Can you work these out from the model? Positions are in its coordinate system, mm. Face numbers are marked on the shaded views. A direction names the side the tool comes from. Coordinates: 2 decimals unless noted, no trailing zeros. Write each loop counter-clockwise with the first axis right and the second up, starting at its lowest first coordinate (ties: lowest second). Pieces come first, ordered by that corner, then holes. Notation, with made-up numbers: (14, 1) - (25, 1) arc R22 cw to (25, 21) - close; hole circle Ø1 at (-15, -21.5). An arc over 180 degrees is marked (long way). One line per question, with ' | ' between items. Start each with the question number.
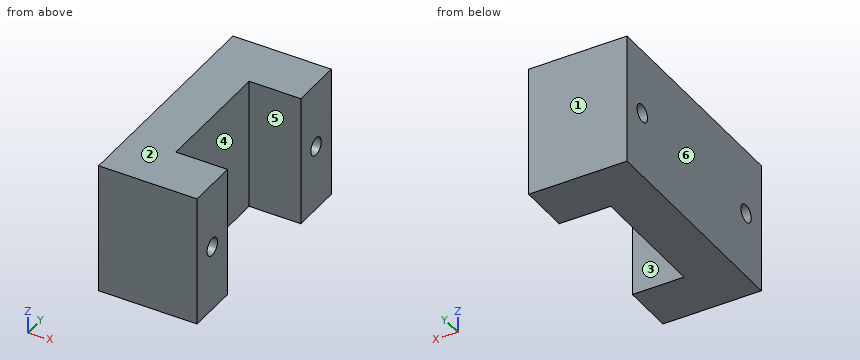
Autodesk Inventor part; units mm, degrees
ref_plane "YZ Plane" through (0, 0, 0) normal (1, 0, 0) x (0, 1, 0)
ref_plane "XZ Plane" through (0, 0, 0) normal (0, 1, 0) x (-1, 0, 0)
ref_plane "XY Plane" through (0, 0, 0) normal (0, 0, 1) x (1, 0, 0)
sketch "Sketch1" plane through (0, 0, 0) normal (1, 0, 0) x (0, 1, 0)
  line L0 (22.6064, 29.4791) -> (-21.3864, 29.4791)
  line L1 (-21.3864, 29.4791) -> (-21.3864, 4.0791)
  line L2 (-21.3864, 4.0791) -> (22.6064, 4.0791)
  line L3 (22.6064, 4.0791) -> (22.6064, 29.4791)
  point P0 (0, 0)
  dimension "d0" = 43.9928
  dimension "d1" = 25.4
extrude "Extrusion1" add sketch "Sketch1" along normal blind 19.05
sketch "Sketch2" plane through (19.05, 0, 0) normal (1, 0, 0) x (0, 0, -1)
  line L0 (-29.4791, 22.6064) -> (-29.4791, -21.3864)
  line L1 (-29.4791, -21.3864) -> (-4.0791, -21.3864)
  line L2 (-4.0791, 22.6064) -> (-29.4791, 22.6064)
  point P0 (0, 0)
  point P1 (-16.7791, 17.6064)
  point P2 (-16.7791, -16.3864)
  dimension "d4" = 0
  dimension "d5" = 12.7
  dimension "d6" = 5
  dimension "d7" = 5
hole "Hole1" at (19.05, 17.6064, 16.7791) at (19.05, -16.3864, 16.7791) direction (-1, 0, 0) diameter 3.4036 end through all
sketch "Sketch3" plane through (0, -21.3864, 29.4791) normal (0, 0, 1) x (1, 0, 0)
  line L0 (19.05, 10) -> (9.05, 10)
  line L1 (9.05, 10) -> (9.05, 33.9928)
  line L2 (9.05, 33.9928) -> (19.05, 33.9928)
  line L3 (19.05, 33.9928) -> (19.05, 10)
  line L4 (19.05, 43.9928) -> (19.05, 0)
  line L5 (0, 43.9928) -> (19.05, 43.9928)
  line L6 (0, 0) -> (19.05, 0)
  point P0 (0, 21.3864)
  dimension "d15" = 0
  dimension "d16" = 10
  dimension "d17" = 10
  dimension "d18" = 10
extrude "Extrusion2" cut sketch "Sketch3" against normal blind 60.325
properties part number "LidarV4MountBack"
(1) If we mould it in two halves opening along Y, with no side actions, what happens to the marked faces 1, 2, 3 and 4? For each: +Y half, -Y half, draft (parallel to the pull), parting line (faces both ways), or undercut.
(2) Which directions (+Z, -Z, +X, -X, +Y, -Y) give clear straight access to the entire face, cutting with the end or side of a thin tool? Please do the marked faces 5 and 6.
(3) If we section it at A-A on x = 16.5: List the corners of the cut face in (y, z) for me.
(4) I'm going to push flat-ended pins straight in: pin 1 (2 mm diameter, centred on y = -3, z = 17, fed in from +X); pin 2 (3 mm diameter, centred on y = 9.5, z = 13.5, fed in from -X); pin 3 (2 mm diameter, centred on y = 17.61, z = 16.78, fed in from +X). Where does each tip first touch, or does it pass through?
(5) If we section it at C-C on z = 6.5: List the corners of the cut face in (x, y) for me, plus the area to 3 significant figures.
(6) If I drill on probe 1 along Y at (x, z) = (18.25, 13.5); probe 2 along Z at (x, y) = (15.75, 17.5); probe 3 along Y at (x, z) = (12.5, 17.75), over which ranges is the centre line in solid material (lowest first)?
(7) If we section it at D-D on x = 7.5: List the corners of the cut face in (y, z) for me, plus the area to 3 significant figures.
(8) If we section it at B-B on y = 17: List the corners of the cut face in (x, z) for me, plus the area to 3 significant figures.
Values:
1) face 1: +Y half | face 2: draft | face 3: undercut | face 4: undercut
2) face 5: +Z, -Z, +X | face 6: +Z, -Z, -X, +Y, -Y
3) outline: (-21.39, 4.08) - (-11.39, 4.08) - (-11.39, 29.48) - (-21.39, 29.48) - close; (12.61, 4.08) - (22.61, 4.08) - (22.61, 29.48) - (12.61, 29.48) - close; hole circle Ø3.4 at (-16.39, 16.78); hole circle Ø3.4 at (17.61, 16.78)
4) pin 1: x = 9.05 | pin 2: x = 0 | pin 3: through
5) outline: (0, -21.39) - (19.05, -21.39) - (19.05, -11.39) - (9.05, -11.39) - (9.05, 12.61) - (19.05, 12.61) - (19.05, 22.61) - (0, 22.61) - close | area: 598 mm2
6) probe 1: -21.39 to -11.39, 12.61 to 22.61 | probe 2: 4.08 to 15.08, 18.48 to 29.48 | probe 3: -21.39 to -17.78, -14.99 to -11.39, 12.61 to 16.21, 19 to 22.61
7) outline: (-21.39, 4.08) - (22.61, 4.08) - (22.61, 29.48) - (-21.39, 29.48) - close; hole circle Ø3.4 at (-16.39, 16.78); hole circle Ø3.4 at (17.61, 16.78) | area: 1,100 mm2
8) outline: (0, 4.08) - (19.05, 4.08) - (19.05, 15.19) - (0, 15.19) - close; (0, 18.37) - (19.05, 18.37) - (19.05, 29.48) - (0, 29.48) - close | area: 423 mm2
